```python
from build123d import *

# Parameters (mm, degrees)
F0_W     = 285.75
F0_H     = 228.6
F1_DEPTH = 19.05
F3_DEPTH = 228.601
F4_SIZE  = 19.04999


# Not quite as in the source:
# - a fillet or chamfer is up to 0.001 mm smaller than in the source, because OpenCascade refuses the exact size


with BuildPart() as f1:
    # F0 (on Right) → F1 (new body)
    with BuildSketch(Plane.YZ):
        Rectangle(F0_W, F0_H)
    extrude(amount=F1_DEPTH)

    # F2 (on face) → F3 (cut, through all)
    with BuildSketch(Plane.XY.offset(114.3)):
        Polygon((0, -142.875), (19.05, -142.875), (0, -131.8764773719), align=None)
        Polygon((19.05, 142.875), (0, 142.875), (19.05, 131.8764773719), align=None)
    extrude(amount=-F3_DEPTH, mode=Mode.SUBTRACT)

    # F4 (size 19.05 in the source; OpenCascade refuses exactly that, so slightly less here)
    f4_edges = [f1.edges().sort_by_distance(p)[0] for p in [
        (19.05, -5.499261, 114.3),
        (19.05, -5.499261, -114.3),
    ]]
    chamfer(f4_edges, length=F4_SIZE)


solid = f1.part
```
Source: CAD feature listing. Evaluate the final solid. Frame: model axes, mm. Coordinates: 2 decimals unless noted, no trailing zeros. Write each loop counter-clockwise with the first axis right and the second up, starting at its lowest first coordinate (ties: lowest second). Pieces come first, ordered by that corner, then holes. Notation, with made-up numbers: M -27,-26.75 L 31,-26.75 A24 cw 31,4.25 Z; hole C 47.5,50.5 d7. An arc over 180 degrees is marked long. Answer as a JSON object with one key per item and string values.
1. Cut plane C-C on x = 10. Output: boundary loops of the cut face in (y, z), plus the area to 3 significant figures.
Evaluation:
{"outline": "M -137.65,-104.3 L 137.1,-104.3 L 137.1,104.3 L -137.65,104.3 Z", "area": "57,300 mm^2"}
2. Contact query for flat-ended pins moving along their axis: P1, Ø4, axis at x = 14, y = -75, coming from the +Z side; P2, Ø4, axis at x = 11, z = 5.5, coming from the +Y side; P3, Ø6, axis at x = 7, y = -112, coming from the +Z side. Output: stop coordinate, or through.
Evaluation:
{"P1": "z = 102.3", "P2": "y = 137.68", "P3": "z = 110.3"}
3. Draft query along Y for faces 1 (the flat face through (9.4, -2, 104.9)), 2 (the flat face through (9.658, -137.453, 1.6)), 3 (the flat face through (9.392, 137.453, 1.6)). Return one class per face: released by +Y, released by -Y, zero draft, split by the parting line, or undercut.
Evaluation:
{"face 1": "zero draft", "face 2": "released by -Y", "face 3": "released by +Y"}
4. Ray query, L1, parallel to Y at x = 11.75, z = 56.5; L2, parallel to Z at x = 3.25, y = -125.5; L3, parallel to Y at x = 17.25, z = 23. Return the intervals inside material, ascending.
Evaluation:
{"L1": "-138.66 to 136.09", "L2": "-111.05 to 111.05", "L3": "-141.84 to 132.92"}
5. Cut plane B-B on z = -49. Output: boundary loops of the cut face in (x, y) (3 decimals).
Evaluation:
{"outline": "M 0,-131.876 L 19.05,-142.875 L 19.05,131.876 L 0,142.875 Z"}
